Part model, mm, in its own coordinate system. Face numbers are marked on the shaded views. A direction names the side the tool comes from. Coordinates: 2 decimals unless noted, no trailing zeros. Order: outer loops, then holes, each group sorted by start corner. A loop starts at its lowest first (then second) coordinate and runs counter-clockwise, first axis right, second up.
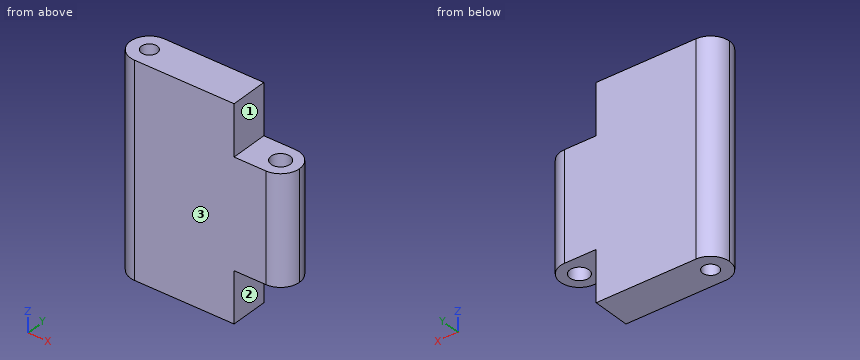
from build123d import *

# Parameters (mm, degrees)
SKETCH1_W           = 13.359057051
SKETCH1_H           = 16.529002792
BOSS_EXTRUDE1_DEPTH = 3
SKETCH2_W           = 4
SKETCH2_H           = 4
CUT_EXTRUDE1_DEPTH  = 22.463278841
FILLET1_R           = 1.5
SKETCH5_R           = 0.625
SKETCH5_R_2         = 0.75
CUT_EXTRUDE3_DEPTH  = 22.463278841
SCALE1_SCALE        = 1.3


with BuildPart() as part:
    # Sketch1 → Boss-Extrude1 (new body)
    with BuildSketch(Plane(origin=(0, 0, 0), x_dir=(1, 0, 0), z_dir=(0, 1, 0))):
        with Locations((6.679528526, 8.264501396)):
            Rectangle(SKETCH1_W, SKETCH1_H)
    extrude(amount=BOSS_EXTRUDE1_DEPTH)

    # Sketch2 → Cut-Extrude1 (cut, through all)
    with BuildSketch(Plane(origin=(0, 3, 0), x_dir=(1, 0, 0), z_dir=(0, 1, 0))):
        with Locations((11.359057051, 14.529002792)):
            Rectangle(SKETCH2_W, SKETCH2_H)
        with Locations((11.359057051, 2)):
            Rectangle(SKETCH2_W, SKETCH2_H)
    extrude(amount=-CUT_EXTRUDE1_DEPTH, mode=Mode.SUBTRACT)

    # Fillet1
    fillet1_edges = [part.edges().sort_by_distance(p)[0] for p in [
        (13.359057051, 0, -8.264501396),
        (13.359057051, 3, -8.264501396),
        (0, 0, -8.264501396),
        (0, 3, -8.264501396),
    ]]
    fillet(fillet1_edges, radius=FILLET1_R - 0.0001)  # a hair under: the kernel refuses the full size

    # Sketch5 → Cut-Extrude3 (cut, through all)
    with BuildSketch(Plane.XY):
        with Locations((1.5, 1.5)):
            Circle(SKETCH5_R)
        with Locations((11.859057051, 1.5)):
            Circle(SKETCH5_R_2)
    extrude(amount=-CUT_EXTRUDE3_DEPTH, mode=Mode.SUBTRACT)


with BuildPart() as part_1:
    # Scale1: scaled about (5.943207595, 1.5, -8.264501396)
    add(part.part.scale(SCALE1_SCALE).moved(Location((-1.782962279, -0.45, 2.479350419))))


solid = part_1.part
Q1. Cut at C-C on x = -0.25. Write the cut outline in (y, z), and give its area (3 significant figures).
Results list:
outline: (-0.4, -19.01) - (0.8, -19.01) - (0.8, 2.48) - (-0.4, 2.48) - close; (2.2, -19.01) - (3.4, -19.01) - (3.4, 2.48) - (2.2, 2.48) - close
area: 51.9 mm2
Q2. Cut at D-D on z = -3.25. Count the separate pieces of the cut face and the enclosed holes in it, and give its area (3 significant figures).
Results list:
separate pieces: 1
enclosed holes: 2
area: 59.4 mm2
Q3. Wall check: line 1 along X through (y, z) = (1.7, -10); line 2 along Z through (x, y) = (10.5, 3.35); line 3 along X through (y, z) = (1.05, -0.75). Give the ranges that are in metal, low to high.
Results list:
line 1: x = -1.77 to -0.62, 0.95 to 12.68, 14.59 to 15.57
line 2: z = -13.81 to -2.72
line 3: x = -1.73 to -0.51, 0.84 to 10.38
Q4. Pin check, flat tips, straight feed: pin 1 Ø1.5 at (y, z) = (3, -2.5) entering from -X; pin 2 Ø2 at (x, y) = (0, 1) entering from -Z; pin 3 Ø1.5 at (x, y) = (0.17, 1.5) entering from +Z; pin 4 Ø2 at (x, y) = (11.5, 3) entering from -Z. Stop position of each tip, or through.
Results list:
pin 1: stops at x = -1.63
pin 2: stops at z = -19.01
pin 3: passes through
pin 4: stops at z = -13.81
Q5. Which spindle directions (+Z, -Z, +X, -X, +Y, -Y) get a long thin tool onto all of the face, cutting with end or side? Do the marked faces 1, 2 and 3. Say none if no direction does.
Results list:
face 1: +Z, +X, +Y, -Y
face 2: -Z, +X, +Y, -Y
face 3: +Z, -Z, +X, -X, -Y
Q6. Cut at B-B on y = 1.05. Write the cut outline in (x, z).
Results list:
outline: (-1.73, -19.01) - (-0.51, -19.01) - (-0.51, 2.48) - (-1.73, 2.48) - close; (0.84, -19.01) - (10.38, -19.01) - (10.38, -13.81) - (12.77, -13.81) - (12.77, -2.72) - (10.38, -2.72) - (10.38, 2.48) - (0.84, 2.48) - close; (14.5, -13.81) - (15.53, -13.81) - (15.53, -2.72) - (14.5, -2.72) - close
